Autodesk Inventor part; units mm, degrees
ref_plane "YZ Plane" through (0, 0, 0) normal (1, 0, 0) x (0, 1, 0)
ref_plane "XZ Plane" through (0, 0, 0) normal (0, 1, 0) x (-1, 0, 0)
ref_plane "XY Plane" through (0, 0, 0) normal (0, 0, 1) x (1, 0, 0)
sketch "スケッチ1" plane through (0, 0, 0) normal (0, 0, 1) x (1, 0, 0)
  circle A0 centre (0, 0) radius 18
  dimension "d0" = 36
extrude "押し出し1" add sketch "スケッチ1" along normal blind 3.25
sketch "スケッチ2" plane through (0, 0, 3.25) normal (0, 0, 1) x (1, 0, 0)
  circle A0 centre (0, 0) radius 6
  point P0 (0, 6)
  point P1 (-6, 0)
  point P2 (0, -6)
  point P3 (6, 0)
  dimension "d3" = 12
  dimension "d6" = 360
hole "穴1" at (0, 6, 3.25) at (-6, 0, 3.25) at (0, -6, 3.25) at (6, 0, 3.25) direction (0, 0, -1) diameter 3.2 end through all counterbore diameter 6.5 counterbore depth 4
sketch "スケッチ3" plane through (0, 0, 0) normal (0, 0, -1) x (-1, 0, 0)
  circle A0 centre (0, 0) radius 8.5
  point P0 (-6.0104, 6.0104)
  point P1 (-6.0104, -6.0104)
  point P2 (6.0104, -6.0104)
  point P3 (6.0104, 6.0104)
  dimension "d15" = 17
  dimension "d50" = 8
  dimension "d18" = 360
hole "穴2" at (6.0104, 6.0104, 0) at (6.0104, -6.0104, 0) at (-6.0104, -6.0104, 0) at (-6.0104, 6.0104, 0) direction (0, 0, 1) diameter 3.2 end through all
sketch "スケッチ4" plane through (0, 0, 0) normal (0, 0, -1) x (-1, 0, 0)
  circle A0 centre (0, 0) radius 3.25
  dimension "d27" = 6.5
extrude "押し出し2" cut sketch "スケッチ4" against normal blind 8
fillet "フィレット1" radius 0.5 8 edges at (-1.25, -3, 1.625) (1.25, -3, 1.625) (3, -1.25, 1.625) (3, 1.25, 1.625) (1.25, 3, 1.625) (-1.25, 3, 1.625) (-3, 1.25, 1.625) (-3, -1.25, 1.625)
sketch "スケッチ5" plane through (0, 0, 3.25) normal (0, 0, 1) x (1, 0, 0)
  circle A0 centre (0, 0) radius 15
  point P0 (0, -15)
  point P1 (10.6066, -10.6066)
  point P2 (15, 0)
  point P3 (10.6066, 10.6066)
  point P4 (0, 15)
  point P5 (-10.6066, 10.6066)
  point P6 (-15, 0)
  point P7 (-10.6066, -10.6066)
  dimension "d31" = 30
  dimension "d34" = 360
hole "穴3" at (0, -15, 3.25) at (10.6066, -10.6066, 3.25) at (15, 0, 3.25) at (10.6066, 10.6066, 3.25) at (0, 15, 3.25) at (-10.6066, 10.6066, 3.25) at (-15, 0, 3.25) at (-10.6066, -10.6066, 3.25) direction (0, 0, -1) diameter 3.2 end through all
sketch "スケッチ6" plane through (0, 0, 3.25) normal (0, 0, 1) x (1, 0, 0)
  circle A0 centre (2.0753, 21.9019) radius 4
  circle A1 centre (-17, 14) radius 4 construction
  circle A2 centre (-3.264, -21.7565) radius 4
  circle A3 centre (0, 0) radius 18
  line L0 (-3.264, -21.7565) -> (0, 0) construction
  circle A4 centre (-20.8592, 6.9924) radius 4 construction
  circle A5 centre (-10.8624, 19.1313) radius 4 construction
  line L1 (-10.8624, 19.1313) -> (0, 0) construction
  line L2 (0, 0) -> (-20.8592, 6.9924) construction
  line L3 (0, 0) -> (2.0753, 21.9019) construction
  arc A6 (-3.8575, -25.7123) -> (2.4526, 25.8841) centre (0, 0) ccw
  circle A7 centre (0, 0) radius 18
  circle A8 centre (-5.8935, 21.1959) radius 4
  circle A9 centre (-10.8278, -19.1509) radius 4
  circle A10 centre (0, 0) radius 22
  point P0 (1.698, 17.9197)
  point P1 (-2.6705, -17.8008)
  point P2 (-1.9091, 21.5489)
  point P3 (-7.1494, -20.8059)
  point P4 (-1.9091, 21.5489)
  point P5 (-4.822, 17.3421)
  point P6 (-8.8591, -15.669)
  point P7 (-7.0459, -20.4537)
  point P8 (-1.9247, 21.9156)
  dimension "d59" = 44
  dimension "d45" = 17
  dimension "d46" = 14
  dimension "d47" = 8
  dimension "d48" = 8
  dimension "d49" = 8
  dimension "d50" = 8
  dimension "d51" = 8
  dimension "d52" = 35
  dimension "d53" = 100
  dimension "d57" = 8
  dimension "d58" = 8
extrude "押し出し3" add sketch "スケッチ6" against normal up to surface (3.25 mm away) contours A10 A2 A3 A0 | A0 A10 | A3 A8 A0 | A2 A10 | A9 A3 A2 picked at (1.947, 20.5476) picked at (-3.0622, -20.4112)
properties part number "s_base5" material "ABS プラスチック"
CAD build for the part. Positions are in the model's coordinates, mm. Round coordinates to 2 decimals unless told otherwise and drop trailing zeros. Loops run counter-clockwise (first coordinate to the right, second up) from the corner with the lowest first, then second, coordinate; pieces in that order, holes last. Notation, with made-up numbers: (-24, 79) - (-3, 79) arc R13 cw to (-3, 93) - close; hole circle Ø2 at (64, 63.25). An arc over 180 degrees is marked (long way). Put each result on its own line as item: value.
1. Slice it at B-B on y = 0. List the corners of the cut face in (x, z).
Geometry check:
outline: (-18, 0) - (-16.6, 0) - (-16.6, 3.25) - (-18, 3.25) - close; (-13.4, 0) - (-9.25, 0) - (-9.25, 3.25) - (-13.4, 3.25) - close; (9.25, 0) - (13.4, 0) - (13.4, 3.25) - (9.25, 3.25) - close; (16.6, 0) - (22, 0) - (22, 3.25) - (16.6, 3.25) - close
2. Two-plate mould, pull along Y, no slides. Class faces 1 (the cylindrical face through (-16.586, 0.208, 1.602)), 2 (the cylindrical face through (21.764, -3.214, 1.648)): released by +Y, released by -Y, zero draft, split by the parting line, or undercut.
Geometry check:
face 1: undercut
face 2: split by the parting line
3. Pin check, flat tips, straight feed: P1, Ø1, axis at y = -14.5, z = 2.5, coming from the -X side; P2, Ø1.5, axis at y = 8, z = 3, coming from the -X side. Stop position of each tip, or through.
Geometry check:
P1: x = -11.31
P2: x = -16.48
4. Slice it at A-A on x = 0. List the corners of the cut face in (y, z).
Geometry check:
outline: (-22, 0) - (-16.6, 0) - (-16.6, 3.25) - (-22, 3.25) - close; (-13.4, 0) - (-9.25, 0) - (-9.25, 3.25) - (-13.4, 3.25) - close; (9.25, 0) - (13.4, 0) - (13.4, 3.25) - (9.25, 3.25) - close; (16.6, 0) - (22, 0) - (22, 3.25) - (16.6, 3.25) - close
5. Slice it at C-C on x = -15. List the corners of the cut face in (y, z).
Geometry check:
outline: (-9.95, 0) - (-1.6, 0) - (-1.6, 3.25) - (-9.95, 3.25) - close; (1.6, 0) - (9.95, 0) - (9.95, 3.25) - (1.6, 3.25) - close
6. Slice it at D-D on z = 1.7. Give the number of separate pieces and of enclosed holes in the cut face, and give its area (3 significant figures).
Geometry check:
separate pieces: 1
enclosed holes: 13
area: 1,050 mm²
7. Wall check: line 1 (X direction, y = 0, z = 2.2); line 2 (Y direction, x = 0, z = 1.9); line 3 (Y direction, x = 10.5, z = 2.6). Give the ranges that are in metal, low to high.
Geometry check:
line 1: -18 to -16.6, -13.4 to -9.25, 9.25 to 13.4, 16.6 to 22
line 2: -22 to -16.6, -13.4 to -9.25, 9.25 to 13.4, 16.6 to 22
line 3: -19.33 to -12.2, -9.01 to 9.01, 12.2 to 19.33
